from build123d import *

# Parameters (mm, degrees)
F0_R          = 44.45
F1_DEPTH      = 25.4
F2_DEPTH      = 1473.2
F3_R          = 31.75
F3_R_2        = 25.4
F4_DEPTH      = 127
F4_DEPTH_BACK = 127


with BuildPart() as f1:
    # F0 (on Front) → F1 (new body)
    with BuildSketch(Plane.XZ):
        Circle(F0_R)
    extrude(amount=F1_DEPTH)

    # F0 (on Front) → F2 (join)
    with BuildSketch(Plane.XZ):
        Circle(F0_R)
    extrude(amount=F2_DEPTH)

    # F3 (on Right) → F4 (join, two sides)
    with BuildSketch(Plane.YZ) as f4_sk:
        with Locations((-736.6, 0)):
            Circle(F3_R)
        with Locations((-736.6, 0)):
            Circle(F3_R_2, mode=Mode.SUBTRACT)
    extrude(amount=F4_DEPTH)
    extrude(f4_sk.sketch, amount=-F4_DEPTH_BACK)


solid = f1.part
CAD build for the part. Positions are in the model's coordinates, mm. A direction names the side the tool comes from. Round coordinates to 2 decimals unless told otherwise and drop trailing zeros. Write each loop counter-clockwise with the first axis right and the second up, starting at its lowest first coordinate (ties: lowest second). Pieces come first, ordered by that corner, then holes. Notation, with made-up numbers: (-38.75, -13.5) -> (17.25, -13.5) arc R19 cw to (17.25, -0.5) -> close; hole circle Ø3 at (16, 87.25). An arc over 180 degrees is marked (long way). Answer as a JSON object with one key per item and string values.
(1) Band-saw the part on C-C, the plane y = -183. List the corners of the cut face in (x, z), then the cut area to 3 significant figures.
Reported:
{"outline": "circle Ø88.9 at (0, 0)", "area": "6,210 mm^2"}
(2) Which spindle directions (+Z, -Z, +X, -X, +Y, -Y) get a long thin tool onto all of the face, cutting with end or side? Do faces 5 (the face through (-127, -750.9, 21.3)), 6 (the face through (-5.79, -726.29, 44.07)), 7 (the face through (-78.38, -707.27, -12.16)). Say none if no direction does.
Reported:
{"face 5": "+Z, -Z, -X, +Y, -Y", "face 6": "none", "face 7": "-X"}
(3) Probe probe 1 along Z at (x, y) = (64, -736.6); probe 2 along Y at (x, z) = (69.5, 0); probe 3 along Y at (x, z) = (-83, 3.5). List the from-to ranges inside material, lowest first. Write a range as [from, to].
Reported:
{"probe 1": "z = [-31.75, -25.4], [25.4, 31.75]", "probe 2": "y = [-768.35, -762], [-711.2, -704.85]", "probe 3": "y = [-768.16, -761.76], [-711.44, -705.04]"}
(4) Band-saw the part on A-A, the plane y = -736.6. List the corners of the cut face in (x, z).
Reported:
{"outline": "(-127, -31.75) -> (-31.11, -31.75) arc R44.45 ccw to (31.11, -31.75) -> (127, -31.75) -> (127, -25.4) -> (36.48, -25.4) arc R44.45 ccw to (36.48, 25.4) -> (127, 25.4) -> (127, 31.75) -> (31.11, 31.75) arc R44.45 ccw to (-31.11, 31.75) -> (-127, 31.75) -> (-127, 25.4) -> (-36.48, 25.4) arc R44.45 ccw to (-36.48, -25.4) -> (-127, -25.4) -> close"}
(5) Pin check, flat tips, straight feed: P1, Ø5, axis at x = -33.5, y = -747, coming from the +Z side; P2, Ø1, axis at x = 18, y = -672.5, coming from the -Z side; P3, Ø3, axis at y = -521.5, z = 16.5, coming from the +X side; P4, Ø1, axis at x = 8.5, z = -21.5, coming from the +Y side. Stop position of each tip, or through.
Reported:
{"P1": "stops at z = 31.86", "P2": "stops at z = -40.86", "P3": "stops at x = 41.84", "P4": "stops at y = 0"}
(6) Band-saw the part on B-B, the plane x = -83. List the corners of the cut face in (y, z), then the cut area to 3 significant figures.
Reported:
{"outline": "circle Ø63.5 at (-736.6, 0); hole circle Ø50.8 at (-736.6, 0)", "area": "1,140 mm^2"}
(7) Two-plate mould, pull along Y, no slides. Class faces 1 (the face through (78.38, -707.27, -12.16)), 2 (the face through (127, -750.9, 21.3)), 3 (the face through (-1, -1473.2, 1)), 4 (the face through (81.105, -712.373, 7.629)): +Y half, -Y half, draft (parallel to the pull), parting line (faces both ways), or undercut.
Reported:
{"face 1": "parting line", "face 2": "draft", "face 3": "-Y half", "face 4": "undercut"}
